Part model, mm, in its own coordinate system. Face numbers are marked on the shaded views. Give positions to 0.01 mm unless a question says otherwise; leave off trailing zeros. Write each loop counter-clockwise with the first axis right and the second up, starting at its lowest first coordinate (ties: lowest second). Pieces come first, ordered by that corner, then holes. Notation, with made-up numbers: (-10.75, -30.75) - (29.25, -30.75) arc R11 ccw to (29.25, -14.75) - close; hole circle Ø3 at (83, 74). An arc over 180 degrees is marked (long way). Answer in a Markdown table with one row per item. Add a question column.
1. Drop a flat-ended pin along its axis: pin 1 Ø1.5 at (x, z) = (5, 117) entering from -Y. Give the stop position or say it passes through.
2. Band-saw the part on B-B on z = 12. Write the cut outline in (x, y), plus the area to 3 significant figures.
3. Band-saw the part on C-C on x = -22.5. Write the cut outline in (y, z).
4. Pull direction Y, two halves, no side cores. Call the marked faces 1, 2 and 3: released by +Y, released by -Y, zero draft, split by the parting line, or undercut.
5. Band-saw the part on A-A on y = 7.75. Write the cut outline in (x, z).
6. Probe line 1 along X through (y, z) = (9, 120); line 2 along Y through (x, z) = (-17.5, 35.5); line 3 along X through (y, z) = (8.5, 163.5). List the from-to ranges inside material, lowest first.
```python
from build123d import *

# Parameters (mm, degrees)
SKETCH1_W               = 80
SKETCH1_H               = 18
BOSS_EXTRUDE1_DEPTH     = 180
CUT_EXTRUDE1_DEPTH      = 1
CUT_EXTRUDE1_DEPTH_BACK = 180


with BuildPart() as part:
    # Sketch1 → Boss-Extrude1 (new body)
    with BuildSketch(Plane.XY):
        with Locations((-11.021069692, 14.824959481)):
            Rectangle(SKETCH1_W, SKETCH1_H)
    extrude(amount=BOSS_EXTRUDE1_DEPTH)

    # Sketch2 → Cut-Extrude1 (cut, two sides)
    with BuildSketch(Plane.XY.offset(180)) as cut_extrude1_sk:
        Polygon((-28.021069692, 5.824959481), (-36.021069692, 13.824959481), (17.978930308, 13.824959481), (9.978930308, 5.824959481), align=None)
    extrude(amount=CUT_EXTRUDE1_DEPTH, mode=Mode.SUBTRACT)
    extrude(cut_extrude1_sk.sketch, amount=-CUT_EXTRUDE1_DEPTH_BACK, mode=Mode.SUBTRACT)


solid = part.part
```
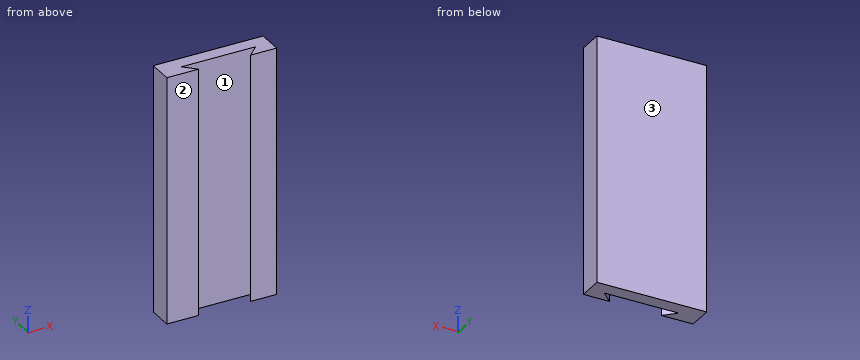
Values:
| question | item | result |
|---|---|---|
| 1 | pin 1 | stops at y = 13.82 |
| 2 | outline | (-51.02, 5.82) - (-28.02, 5.82) - (-36.02, 13.82) - (17.98, 13.82) - (9.98, 5.82) - (28.98, 5.82) - (28.98, 23.82) - (-51.02, 23.82) - close |
| 2 | area | 1,070 mm² |
| 3 | outline | (13.82, 0) - (23.82, 0) - (23.82, 180) - (13.82, 180) - close |
| 4 | face 1 | undercut |
| 4 | face 2 | released by -Y |
| 4 | face 3 | released by +Y |
| 5 | outline | (-51.02, 0) - (-29.95, 0) - (-29.95, 180) - (-51.02, 180) - close; (11.9, 0) - (28.98, 0) - (28.98, 180) - (11.9, 180) - close |
| 6 | line 1 | x = -51.02 to -31.2, 13.15 to 28.98 |
| 6 | line 2 | y = 13.82 to 23.82 |
| 6 | line 3 | x = -51.02 to -30.7, 12.65 to 28.98 |
